Autodesk Inventor part; units mm, degrees
ref_plane "YZ Plane" through (0, 0, 0) normal (1, 0, 0) x (0, 1, 0)
ref_plane "XZ Plane" through (0, 0, 0) normal (0, 1, 0) x (-1, 0, 0)
ref_plane "XY Plane" through (0, 0, 0) normal (0, 0, 1) x (1, 0, 0)
sketch "Boceto1" plane through (0, 0, 0) normal (0, 0, 1) x (1, 0, 0)
  circle A0 centre (0, 0) radius 25
  circle A1 centre (0, 0) radius 4
  circle A2 centre (0, 0) radius 11
  dimension "d0" = 50
  dimension "d3" = 8
  dimension "d34" = 22
extrude "Extrusión1" add sketch "Boceto1" along normal blind 10 contours A0 | A2
sketch "Boceto5" plane through (0, 0, 10) normal (0, 0, 1) x (1, 0, 0)
  circle A0 centre (0, 0) radius 4
  circle A1 centre (0, 0) radius 15
  dimension "d15" = 8
  dimension "d16" = 30
extrude "Extrusión5" add sketch "Boceto5" along normal blind 40
sketch "Boceto6" plane through (0, 0, 50) normal (0, 0, 1) x (1, 0, 0)
  circle A0 centre (0, 0) radius 4
  circle A1 centre (0, 0) radius 25
  circle A2 centre (0, 0) radius 4
  circle A3 centre (0, 0) radius 11
  dimension "d22" = 50
  dimension "d30" = 8
  dimension "d31" = 22
extrude "Extrusión13" add sketch "Boceto6" along normal blind 10 contours A1 | A3
sketch "Boceto17" plane through (0, 0, 10) normal (0, 0, 1) x (1, 0, 0)
  circle A0 centre (0, 20.0085) radius 1.5
  point P0 (0, 0)
  dimension "d102" = 3
extrude "Extrusión14" cut sketch "Boceto17" against normal blind 10
properties part number "carrete"
Verification items for the finished model (mm, model axes). A direction names the side the tool comes from. Coordinates: 2 decimals unless noted, no trailing zeros. Write each loop counter-clockwise with the first axis right and the second up, starting at its lowest first coordinate (ties: lowest second). Pieces come first, ordered by that corner, then holes. Notation, with made-up numbers: M -17.75,31 L 0.25,31 A9 ccw 0.25,46 Z; hole C -21.75,46 d5. An arc over 180 degrees is marked long. One line per question, with ' | ' between items.
1) Release check for a two-part mould opening along Y. For faces 3 (the face through (11, -11, 50)), 4 (the face through (23.846, -7.509, 54.93)), 5 (the face through (0.81, 21.27, 5.07)) record: +Y half, -Y half, draft (parallel to the pull), parting line (faces both ways), or undercut.
Solutions:
face 3: draft | face 4: parting line | face 5: undercut
2) Sectioned sample at D-D on y = 7. Record the cut outline in (x, z), then the cut area to 3 significant figures.
Solutions:
outline: M -24,0 L 24,0 L 24,10 L 13.27,10 L 13.27,50 L 24,50 L 24,60 L -24,60 L -24,50 L -13.27,50 L -13.27,10 L -24,10 Z | area: 2,020 mm^2
3) Access from +Z, -Z, +X, -X, +Y, -Y to the whole of each face (thin tool, end or side, straight path). Record for faces 1 (the face through (23.846, -7.509, 4.93)), 2 (the face through (-14.985, -0.66, 29.72)).
Solutions:
face 1: +Z, -Z | face 2: none
4) Depth check by flat-ended pin: pin 1 Ø8 at (x, y) = (1, 2.5) entering from -Z; pin 2 Ø5 at (x, z) = (3, 16) entering from +Y; pin 3 Ø5 at (x, z) = (-6.5, 23.5) entering from -Y; pin 4 Ø12 at (y, z) = (8.5, 36) entering from -X. Enter the tip coordinate at first touch or a pass-through.
Solutions:
pin 1: z = 0 | pin 2: y = 14.99 | pin 3: y = -14.46 | pin 4: x = -14.79
5) Sectioned sample at B-B on y = 0. Record the cut outline in (x, z), then the cut area to 3 significant figures.
Solutions:
outline: M -25,0 L -4,0 L -4,60 L -25,60 L -25,50 L -15,50 L -15,10 L -25,10 Z; M 4,0 L 25,0 L 25,10 L 15,10 L 15,50 L 25,50 L 25,60 L 4,60 Z | area: 1,720 mm^2
6) Sectioned sample at C-C on z = 16. Record the cut outline in (x, y).
Solutions:
outline: C 0,0 d30; hole C 0,0 d8
7) Material ranges on L1, parallel to Y at x = 0, z = 3.5; L2, parallel to Z at x = 18.5, y = -13.5; L3, parallel to Y at x = 0, z = 38, recorded low to high.
Solutions:
L1: -25 to -4, 4 to 18.51, 21.51 to 25 | L2: 0 to 10, 50 to 60 | L3: -15 to -4, 4 to 15
8) Sectioned sample at A-A on x = 0. Record the cut outline in (y, z), then the cut area to 3 significant figures.
Solutions:
outline: M -25,0 L -4,0 L -4,60 L -25,60 L -25,50 L -15,50 L -15,10 L -25,10 Z; M 4,0 L 18.51,0 L 18.51,10 L 15,10 L 15,50 L 25,50 L 25,60 L 4,60 Z; M 21.51,0 L 25,0 L 25,10 L 21.51,10 Z | area: 1,690 mm^2
